Model file for the job. Use its own axes, mm. A direction names the side the tool comes from. Give positions to 0.01 mm unless a question says otherwise; leave off trailing zeros. Write each loop counter-clockwise with the first axis right and the second up, starting at its lowest first coordinate (ties: lowest second). Pieces come first, ordered by that corner, then holes.
```python
from build123d import *

# Parameters (mm, degrees)
SKETCH1_W           = 50
SKETCH1_H           = 30
BOSS_EXTRUDE1_DEPTH = 10
SKETCH2_R           = 7.5
CUT_EXTRUDE1_DEPTH  = 10
SKETCH3_W           = 50
SKETCH3_H           = 30
BOSS_EXTRUDE2_DEPTH = 40
SKETCH4_R           = 10.5
CUT_EXTRUDE2_DEPTH  = 40
SKETCH5_W           = 50
SKETCH5_H           = 30
BOSS_EXTRUDE3_DEPTH = 5
SKETCH6_W           = 50
SKETCH6_H           = 30
BOSS_EXTRUDE4_DEPTH = 5
SKETCH7_R           = 10
BOSS_EXTRUDE5_DEPTH = 10


with BuildPart() as part:
    # Sketch1 → Boss-Extrude1 (new body)
    with BuildSketch(Plane.XY):
        with Locations((-25, 15)):
            Rectangle(SKETCH1_W, SKETCH1_H)
    extrude(amount=BOSS_EXTRUDE1_DEPTH)

    # Sketch2 → Cut-Extrude1 (cut)
    with BuildSketch(Plane.XY.offset(10)):
        with Locations((-37.5, 15)):
            Circle(SKETCH2_R)
        with Locations((-12.5, 15)):
            Circle(SKETCH2_R)
    extrude(amount=-CUT_EXTRUDE1_DEPTH, mode=Mode.SUBTRACT)

    # Sketch3 → Boss-Extrude2 (add)
    with BuildSketch(Plane.XY.offset(10)):
        with Locations((-25, 15)):
            Rectangle(SKETCH3_W, SKETCH3_H)
    extrude(amount=BOSS_EXTRUDE2_DEPTH)

    # Sketch4 → Cut-Extrude2 (cut)
    with BuildSketch(Plane.XY.offset(50)):
        with Locations((-37.5, 15)):
            Circle(SKETCH4_R)
        with Locations((-12.5, 15)):
            Circle(SKETCH4_R)
    extrude(amount=-CUT_EXTRUDE2_DEPTH, mode=Mode.SUBTRACT)

    # Sketch5 → Boss-Extrude3 (add)
    with BuildSketch(Plane(origin=(0, 0, 0), x_dir=(0, 0, -1), z_dir=(1, 0, 0))):
        with Locations((-25, 15)):
            Rectangle(SKETCH5_W, SKETCH5_H)
    extrude(amount=BOSS_EXTRUDE3_DEPTH)

    # Sketch6 → Boss-Extrude4 (add)
    with BuildSketch(Plane.ZY.offset(50)):
        with Locations((25, 15)):
            Rectangle(SKETCH6_W, SKETCH6_H)
    extrude(amount=BOSS_EXTRUDE4_DEPTH)

    # Sketch7 → Boss-Extrude5 (add)
    with BuildSketch(Plane(origin=(0, 30, 0), x_dir=(1, 0, 0), z_dir=(0, 1, 0))):
        with Locations(Location((-25, -25, 0), (0, 0, 180))):
            Circle(SKETCH7_R)
    extrude(amount=BOSS_EXTRUDE5_DEPTH)


solid = part.part
```
1. Slice it at D-D, the plane x = -25. Write the cut outline in (y, z).
Calculated:
outline: (0, 0) - (30, 0) - (30, 15) - (40, 15) - (40, 35) - (30, 35) - (30, 50) - (0, 50) - close
2. Slice it at C-C, the plane z = 25. Write the cut outline in (x, y).
Calculated:
outline: (-55, 0) - (5, 0) - (5, 30) - (-15, 30) - (-15, 40) - (-35, 40) - (-35, 30) - (-55, 30) - close; hole circle Ø21 at (-37.5, 15); hole circle Ø21 at (-12.5, 15)
3. Probe probe 1 along Y at (x, z) = (-37.5, 4.5); probe 2 along X at (y, z) = (22, 25); probe 3 along X at (y, z) = (14, 46). List the from-to ranges inside material, lowest first.
Calculated:
probe 1: y = 0 to 7.5, 22.5 to 30
probe 2: x = -55 to -45.33, -29.67 to -20.33, -4.67 to 5
probe 3: x = -55 to -47.95, -27.05 to -22.95, -2.05 to 5
4. Pull direction X, two halves, no side cores. Call faces 4 (the cylindrical face through (-48, 15, 30)), 5 (the flat face through (-25, 30, 14)), 6 (the flat face through (5, 15, 25)): +X half, -X half, draft (parallel to the pull), parting line (faces both ways), or undercut.
Calculated:
face 4: undercut
face 5: draft
face 6: +X half
5. Slice it at B-B, the plane y = 15. Write the cut outline in (x, z).
Calculated:
outline: (-55, 0) - (-45, 0) - (-45, 10) - (-48, 10) - (-48, 50) - (-55, 50) - close; (-30, 0) - (-20, 0) - (-20, 10) - (-23, 10) - (-23, 50) - (-27, 50) - (-27, 10) - (-30, 10) - close; (-5, 0) - (5, 0) - (5, 50) - (-2, 50) - (-2, 10) - (-5, 10) - close
6. Slice it at A-A, the plane x = -37.5. Write the cut outline in (y, z).
Calculated:
outline: (0, 0) - (7.5, 0) - (7.5, 10) - (4.5, 10) - (4.5, 50) - (0, 50) - close; (22.5, 0) - (30, 0) - (30, 50) - (25.5, 50) - (25.5, 10) - (22.5, 10) - close
7. Which spindle directions (+Z, -Z, +X, -X, +Y, -Y) get a long thin tool onto all of the face, cutting with end or side? Do faces 1 (the flat face through (-20, 17, 10)), 2 (the cylindrical face through (-34.54, 34.93, 28)), 3 (the flat face through (-55, 15, 25)). Say none if no direction does.
Calculated:
face 1: +Z
face 2: +Y
face 3: +Z, -Z, -X, +Y, -Y
8. Pin check, flat tips, straight feed: P1, Ø6, axis at x = -22.5, z = 7.5, coming from the +Y side; P2, Ø12, axis at x = -37.5, y = 15, coming from the -Z side; P3, Ø3, axis at x = -30.5, y = 13.5, coming from the +Z side. Stop position of each tip, or through.
Calculated:
P1: stops at y = 30
P2: passes through
P3: stops at z = 10
